Source: CAD feature listing. Evaluate the final solid. Frame: model axes, mm. Give positions to 0.01 mm unless a question says otherwise; leave off trailing zeros. Loops run counter-clockwise (first coordinate to the right, second up) from the corner with the lowest first, then second, coordinate; pieces in that order, holes last. Notation, with made-up numbers: (-4.75, -27.75) -> (6.25, -27.75) arc R31 ccw to (6.25, -0.75) -> close; hole circle Ø10 at (-28.5, 79.5). An arc over 180 degrees is marked (long way). Answer as a JSON object with one key per item and string values. Group by question number.
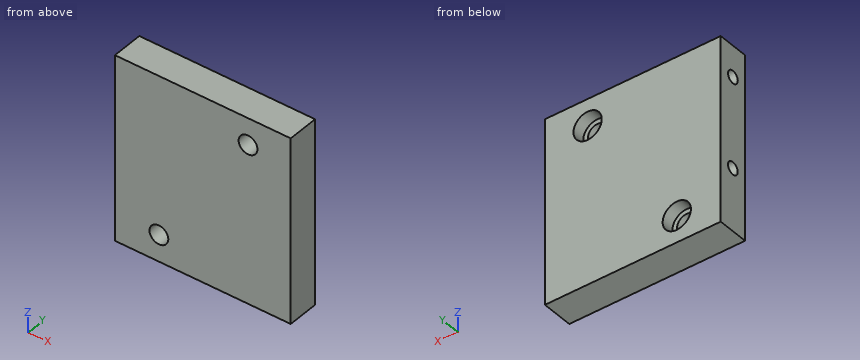
from build123d import *

# Parameters (mm, degrees)
SKETCH_1_W          = 28
SKETCH_1_H          = 29.5
EXTRUDE_1_DEPTH     = 5
SKETCH_1_20_R       = 1.5
CUT_EXTRUDE_1_DEPTH = 41.978652979
CUT_EXTRUDE_START   = 5
SKETCH_1_21_R       = 2.25
CUT_EXTRUDE_2_DEPTH = 2
SKETCH_4_R          = 1
CUT_EXTRUDE_3_DEPTH = 4


with BuildPart() as part:
    # 草图1 → 凸台-拉伸1 (new body)
    with BuildSketch(Plane(origin=(0, 0, 0), x_dir=(1, 0, 0), z_dir=(0, 1, 0))):
        with Locations((-14, -14.75)):
            Rectangle(SKETCH_1_W, SKETCH_1_H)
    extrude(amount=EXTRUDE_1_DEPTH)

    # 草图1<20> → 切除-拉伸1 (cut, through all)
    with BuildSketch(Plane(origin=(0, 0, 0), x_dir=(1, 0, 0), z_dir=(0, 1, 0))):
        with Locations(Location((-21, -4.25, 0), (0, 0, 270))):
            Circle(SKETCH_1_20_R)
        with Locations(Location((-6.8, -25.25, 0), (0, 0, 270))):
            Circle(SKETCH_1_20_R)
    extrude(amount=CUT_EXTRUDE_1_DEPTH, mode=Mode.SUBTRACT)

    # 草图1<21> → 切除-拉伸2 (cut)
    with BuildSketch(Plane(origin=(0, 0, 0), x_dir=(1, 0, 0), z_dir=(0, 1, 0)).offset(CUT_EXTRUDE_START)):
        with Locations(Location((-21, -4.25, 0), (0, 0, 270))):
            Circle(SKETCH_1_21_R)
        with Locations(Location((-6.8, -25.25, 0), (0, 0, 270))):
            Circle(SKETCH_1_21_R)
    extrude(amount=-CUT_EXTRUDE_2_DEPTH, mode=Mode.SUBTRACT)

    # 草图4 → 切除-拉伸3 (cut)
    with BuildSketch(Plane.ZY.offset(28)):
        with Locations((10, 2.5)):
            Circle(SKETCH_4_R)
        with Locations((24.5, 2.5)):
            Circle(SKETCH_4_R)
    extrude(amount=-CUT_EXTRUDE_3_DEPTH, mode=Mode.SUBTRACT)


solid = part.part
(1) Section query D-D on x = -26. Return the cut outline in (y, z), plus the area to 3 significant figures.
(2) Material intervals for line 1 (X direction, y = 4.35, z = 25.25); line 2 (Y direction, x = -25.2, z = 24.5); line 3 (Z direction, x = -6.8, y = 1.3), sorted ascending. Write a range as from..to.
(3) Section query A-A on x = -21. Return the cut outline in (y, z).
(4) First-contact query: pin 1 (0.6 mm diameter, centred on y = 2.5, z = 24, fed in from -X); pin 2 (2 mm diameter, centred on x = -18, y = 4, fed in from -Z); pin 3 (2.5 mm diameter, centred on x = -21, z = 4.25, fed in from +Y); pin 4 (3.5 mm diameter, centred on x = -7, z = 25.5, fed in from +Y). Flat tips, straight axial feed; report the tip coordinate or a pass-through.
(5) Section query B-B on y = 2.5. Return the cut outline in (x, z).
(6) Section query C-C on z = 3.75. Return the cut outline in (x, y), plus the area to 3 significant figures.
Result:
{
 "1": {"outline": "(0, 0) -> (5, 0) -> (5, 29.5) -> (0, 29.5) -> close; hole circle Ø2 at (2.5, 10); hole circle Ø2 at (2.5, 24.5)", "area": "141 mm²"},
 "2": {"line 1": "-28..-9.05, -4.55..0", "line 2": "0..1.5, 3.5..5", "line 3": "0..23.75, 26.75..29.5"},
 "3": {"outline": "(0, 0) -> (5, 0) -> (5, 2) -> (3, 2) -> (3, 2.75) -> (0, 2.75) -> close; (0, 5.75) -> (3, 5.75) -> (3, 6.5) -> (5, 6.5) -> (5, 29.5) -> (0, 29.5) -> close"},
 "4": {"pin 1": "x = -24", "pin 2": "z = 0", "pin 3": "through", "pin 4": "y = 3"},
 "5": {"outline": "(-28, 0) -> (0, 0) -> (0, 29.5) -> (-28, 29.5) -> (-28, 25.5) -> (-24, 25.5) -> (-24, 23.5) -> (-28, 23.5) -> (-28, 11) -> (-24, 11) -> (-24, 9) -> (-28, 9) -> close; hole circle Ø3 at (-21, 4.25); hole circle Ø3 at (-6.8, 25.25)"},
 "6": {"outline": "(-28, 0) -> (-22.41, 0) -> (-22.41, 3) -> (-23.19, 3) -> (-23.19, 5) -> (-28, 5) -> close; (-19.59, 0) -> (0, 0) -> (0, 5) -> (-18.81, 5) -> (-18.81, 3) -> (-19.59, 3) -> close", "area": "123 mm²"}
}
